Could you check a few things on this model? Use its own coordinates, in mm. Give positions to 0.01 mm unless a question says otherwise; leave off trailing zeros. Loops run counter-clockwise (first coordinate to the right, second up) from the corner with the lowest first, then second, coordinate; pieces in that order, holes last. Notation, with made-up numbers: M 44,-22 L 90,-22 A16 ccw 90,-2 Z; hole C 15,37.25 d9. An arc over 180 degrees is marked long. Answer in a Markdown table with one row per item. Add a question column.
1. If we section it at A-A on x = 15.5: List the corners of the cut face in (y, z) for me.
2. Thinking about a two-plate mould opening in Y: for faces 1 (the flat face through (0, 0, 0)), 2 (the cylindrical face through (60.833, -0.867, -3.905)), which applies, released by +Y, released by -Y, zero draft, split by the parting line, or undercut?
3. I'm going to push flat-ended pins straight in: pin 1 Ø3 at (x, z) = (55.5, 2.5) entering from +Y; pin 2 Ø2 at (x, z) = (48.5, -2) entering from -Y; pin 3 Ø3 at (x, z) = (16.5, 2) entering from -Y. Where does each tip first touch, or does it pass through?
4. I need wall thicknesses on line 1 along Z through (x, y) = (73, -0.25); line 2 along Z through (x, y) = (115, 2.5); line 3 along X through (y, z) = (-1.25, -3.5). Which ranges of each line are inside material? Lowest first, please. Write a range as from..to.
Autodesk Inventor part; units mm, degrees
ref_plane "Startebene" through (0, 0, 0) normal (1, 0, 0) x (0, 1, 0)
ref_plane "XZ Plane" through (0, 0, 0) normal (0, 1, 0) x (-1, 0, 0)
ref_plane "XY Plane" through (0, 0, 0) normal (0, 0, 1) x (1, 0, 0)
sketch "Hauptskizze" plane through (0, 0, 0) normal (0, 0, 1) x (1, 0, 0)
  line L0 (0, 0) -> (120, 0)
  line L1 (0, 0) -> (0, 4)
  line L2 (120, 4) -> (120, 0)
  line L3 (0, 4) -> (120, 4)
  dimension "d3" = 8
revolve "Umdrehung1" add sketch "Hauptskizze" angle 360 about axis through (0, 0, 0) along (1, 0, 0)
chamfer "Fase3" distance 0.5 angle 45 1 edges at (0, -4, 0) measured on face at (80, 3.987, -0.3219)
chamfer "Fase2" distance 0.5 angle 45 1 edges at (120, -4, 0) measured on face at (80.1667, 3.987, -0.3219)
properties part number "Welle 8x120mm" material "Steel"
Results:
| question | item | result |
|---|---|---|
| 1 | outline | C 0,0 d8 |
| 2 | face 1 | zero draft |
| 2 | face 2 | split by the parting line |
| 3 | pin 1 | y = 3.87 |
| 3 | pin 2 | y = -3.87 |
| 3 | pin 3 | y = -3.97 |
| 4 | line 1 | -3.99..3.99 |
| 4 | line 2 | -3.12..3.12 |
| 4 | line 3 | 0.22..119.78 |
